Geometry: final body of the model. Coordinates: model frame, mm. Face numbers are marked on the shaded views. Give positions to 0.01 mm unless a question says otherwise; leave off trailing zeros. Order: outer loops, then holes, each group sorted by start corner. A loop starts at its lowest first (then second) coordinate and runs counter-clockwise, first axis right, second up. Notation, with made-up numbers: (34.25, 36) - (39.25, 36) arc R33 cw to (39.25, 64) - close; hole circle Ø9 at (60.25, -11). An arc over 180 degrees is marked (long way). Use one line per item in the form item = value.
Autodesk Inventor part; units mm, degrees
ref_plane "Work Plane1" through (0, -0.3986, 8.06) normal (0, 0, 1) x (1, 0, 0)
ref_plane "Work Plane2" through (0, -0.3986, -2.17) normal (0, 0, -1) x (-1, 0, 0)
ref_plane "YZ Plane" through (0, 0, 0) normal (1, 0, 0) x (0, 1, 0)
sketch "Sketch1" plane through (0, 0, 0) normal (0, 0, 1) x (1, 0, 0)
  circle A0 centre (0, -0.3986) radius 11.95
  point P0 (0, 0)
  dimension "d0" = 23.9
extrude "Extrusion1" add sketch "Sketch1" along normal blind 5.89
ref_plane "Work Plane1" through (0, -0.3986, 8.06) normal (0, 0, 1) x (1, 0, 0)
sketch "Sketch2" plane through (0, -0.3986, 8.06) normal (0, 0, 1) x (1, 0, 0)
  circle A0 centre (0, 0) radius 8
  point P0 (0, 0.3986)
  dimension "d4" = 16
sketch "Sketch5" plane through (0, -0.3986, 5.89) normal (0, 0, 1) x (1, 0, 0)
  circle A0 centre (0, 0) radius 11.95
  point P0 (0, 0.3986)
  dimension "d5" = 23.9
loft "Loft1" add profiles "Sketch2", "Sketch5"
ref_plane "Work Plane2" through (0, -0.3986, -2.17) normal (0, 0, -1) x (-1, 0, 0)
sketch "Sketch6" plane through (0, -0.3986, -2.17) normal (0, 0, -1) x (-1, 0, 0)
  circle A0 centre (0, 0) radius 8
  point P0 (0, 0.3986)
  dimension "d11" = 16
sketch "Sketch7" plane through (0, -0.3986, 0) normal (0, 0, -1) x (-1, 0, 0)
  circle A0 centre (0, 0) radius 11.95
  point P0 (0, 0.3986)
  dimension "d12" = 23.9
loft "Loft2" add profiles "Sketch6", "Sketch7"
sketch "Sketch8" plane through (0, -0.3986, 8.06) normal (0, 0, 1) x (1, 0, 0)
  circle A0 centre (0, 0) radius 2.5
  point P0 (0, 0.3986)
  dimension "d17" = 5
extrude "Extrusion2" cut sketch "Sketch8" against normal blind 15
properties part number "RUEDA"
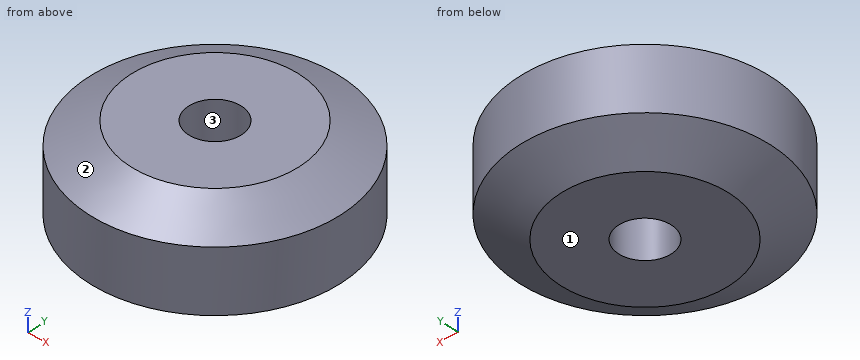
(1) Cut plane C-C on z = 4. Output: boundary loops of the cut face in (x, y), plus the area to 3 significant figures.
Computed values:
outline = circle Ø23.9 at (0, -0.4); hole circle Ø5 at (0, -0.4)
area = 429 mm²
(2) Cut plane B-B on z = -1. Output: boundary loops of the cut face in (x, y), plus the area to 3 significant figures.
Computed values:
outline = circle Ø20.26 at (0, -0.4); hole circle Ø5 at (0, -0.4)
area = 303 mm²
(3) Cut plane A-A on x = 0. Output: boundary loops of the cut face in (y, z), plus the area to 3 significant figures.
Computed values:
outline = (-12.35, 0) - (-8.4, -2.17) - (-2.9, -2.17) - (-2.9, 8.06) - (-8.4, 8.06) - (-12.35, 5.89) - close; (2.1, -2.17) - (7.6, -2.17) - (11.55, 0) - (11.55, 5.89) - (7.6, 8.06) - (2.1, 8.06) - close
area = 176 mm²
(4) Pull-direction query (Y, two-part tool) for the marked faces 1, 2 and 3; classes: released by +Y, released by -Y, zero draft, split by the parting line, or undercut.
Computed values:
face_1 = zero draft
face_2 = split by the parting line
face_3 = undercut
(5) Ray query, line 1 along Y through (x, z) = (0, 3.5); line 2 along X through (y, z) = (-0.5, 1.25); line 3 along X through (y, z) = (1.25, 4). Return the intervals inside material, ascending.
Computed values:
line_1 = -12.35 to -2.9, 2.1 to 11.55
line_2 = -11.95 to -2.5, 2.5 to 11.95
line_3 = -11.84 to -1.88, 1.88 to 11.84
(6) Contact query for flat-ended pins moving along their axis: pin 1 Ø5 at (y, z) = (-5.5, 4.5) entering from +X; pin 2 Ø2 at (x, y) = (8.5, -3) entering from +Z; pin 3 Ø5 at (y, z) = (-4, 2) entering from -X; pin 4 Ø6 at (x, z) = (9.5, 3.5) entering from -Y. Output: stop coordinate, or through.
Computed values:
pin_1 = 11.66
pin_2 = 8.06
pin_3 = -11.9
pin_4 = -10.43
